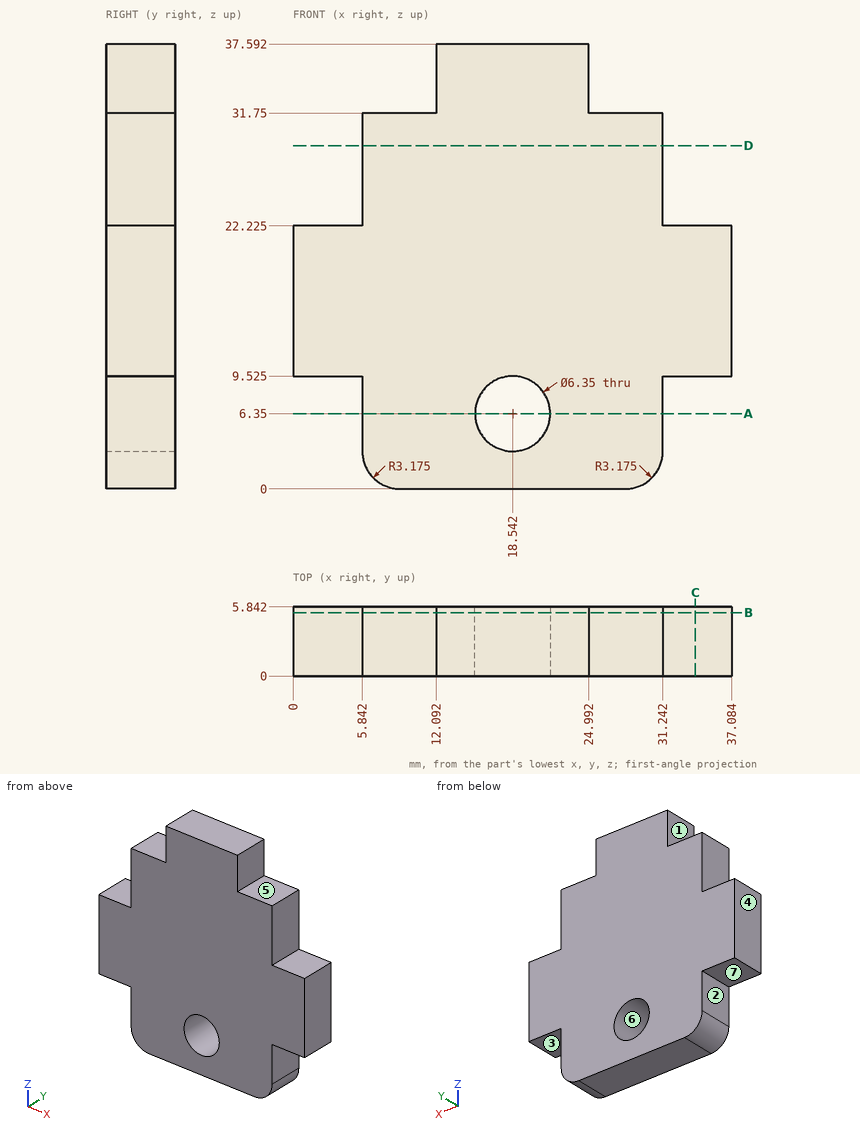
Here's the drawing with two shaded views (mm, measured from the low corner). I have some questions. A direction names the side the tool comes from. Coordinates: 2 decimals unless noted, no trailing zeros. Loops run counter-clockwise (first coordinate to the right, second up) from the corner with the lowest first, then second, coordinate; pieces in that order, holes last.
Item 1: If we mould it in two halves opening along Z, with no side actions, what happens to the marked faces 4, 5, 6 and 7? For each: released by +Z, released by -Z, zero draft, split by the parting line, or undercut.
Answers below:
face 4: zero draft
face 5: released by +Z
face 6: undercut
face 7: released by -Z
Item 2: Suppose I cut it at B-B (y = 5.35). Please give me the cut outline in (x, z) (3 decimals), then the cut area to 3 significant figures.
Answers below:
outline: (0, 9.525) - (5.842, 9.525) - (5.842, 3.175) arc R3.175 ccw to (9.017, 0) - (28.067, 0) arc R3.175 ccw to (31.242, 3.175) - (31.242, 9.525) - (37.084, 9.525) - (37.084, 22.225) - (31.242, 22.225) - (31.242, 31.75) - (24.992, 31.75) - (24.992, 37.592) - (12.092, 37.592) - (12.092, 31.75) - (5.842, 31.75) - (5.842, 22.225) - (0, 22.225) - close; hole circle Ø6.35 at (18.542, 6.35)
area: 994 mm2
Item 3: I'm going to push flat-ended pins straight in: pin 1 (1.8 mm diameter, centred on x = 8.5, y = 2.5, fed in from +Z); pin 2 (1.8 mm diameter, centred on x = 34.5, y = 4, fed in from +Z) (3 decimals); pin 3 (1.5 mm diameter, centred on y = 3, z = 5, fed in from -X). Where does each tip first touch, or does it pass through?
Answers below:
pin 1: stops at z = 31.75
pin 2: stops at z = 22.225
pin 3: stops at x = 5.84
Item 4: Please list where these lines run through material, in increasing order: L1, parallel to Z at x = 9, y = 1.85; L2, parallel to Z at x = 35, y = 2.7 (3 decimals); L3, parallel to Z at x = 19.5, y = 1.15.
Answers below:
L1: z = 0 to 31.75
L2: z = 9.525 to 22.225
L3: z = 0 to 3.32, 9.38 to 37.59
Item 5: Suppose I cut it at C-C (x = 34). Please give me the cut outline in (y, z) (3 decimals), then the cut area to 3 significant figures.
Answers below:
outline: (0, 9.525) - (5.842, 9.525) - (5.842, 22.225) - (0, 22.225) - close
area: 74.2 mm2
Item 6: Which directions (+Z, -Z, +X, -X, +Y, -Y) give clear straight access to the entire face, cutting with the end or side of a thin tool? Please do the marked faces 1, 2 and 3.
Answers below:
face 1: +Z, -X, +Y, -Y
face 2: -Z, -X, +Y, -Y
face 3: -Z, +X, +Y, -Y
Item 7: Suppose I cut it at D-D (z = 29). Please give me the cut outline in (x, y), then the cut area to 3 significant figures.
Answers below:
outline: (5.84, 0) - (31.24, 0) - (31.24, 5.84) - (5.84, 5.84) - close
area: 148 mm2
Item 8: Suppose I cut it at A-A (z = 6.35). Please give me the cut outline in (x, y).
Answers below:
outline: (5.84, 0) - (15.37, 0) - (15.37, 5.84) - (5.84, 5.84) - close; (21.72, 0) - (31.24, 0) - (31.24, 5.84) - (21.72, 5.84) - close
